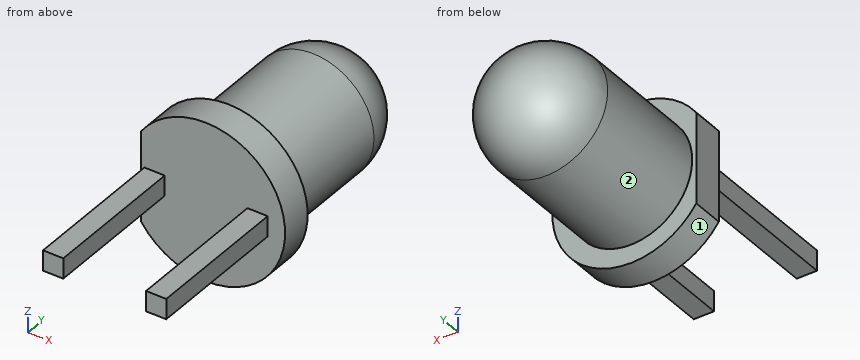
from build123d import *

# Parameters (mm, degrees)
ESQUISSE2_W             = 0.5
ESQUISSE2_H             = 0.5
BOSS_EXTRU_1_DEPTH      = 3.6
ESQUISSE3_W             = 1
ESQUISSE3_H             = 4
ENL_V_MAT_EXTRU_1_DEPTH = 6.3


with BuildPart() as part:
    # Esquisse1 → Révolution1 (revolve)
    with BuildSketch(Plane.XY):
        with BuildLine():
            Line((0, 0), (-1.95, 0))
            Line((-1.95, 0), (-1.95, 0.8))
            Line((-1.95, 0.8), (-1.5, 0.8))
            Line((-1.5, 0.8), (-1.5, 3.8))
            ThreePointArc((-1.5, 3.8), (-1.060660172, 4.860660172), (0, 5.3))
            Line((0, 5.3), (0, 0))
        make_face()
    revolve(axis=Axis((0, 5.3, 0), (0, -1, 0)))

    # Esquisse2 → Boss.-Extru.1 (add)
    with BuildSketch(Plane.XZ):
        with Locations((-1.27, 0)):
            Rectangle(ESQUISSE2_W, ESQUISSE2_H)
        with Locations((1.27, 0)):
            Rectangle(ESQUISSE2_W, ESQUISSE2_H)
    extrude(amount=BOSS_EXTRU_1_DEPTH)

    # Esquisse3 → Enlèv. mat.-Extru.1 (cut, through all)
    with BuildSketch(Plane.XZ):
        with Locations((-2.1, 0)):
            Rectangle(ESQUISSE3_W, ESQUISSE3_H)
    extrude(amount=-ENL_V_MAT_EXTRU_1_DEPTH, mode=Mode.SUBTRACT)


solid = part.part
The listing builds one solid part. Answer for the finished solid, in the listing's coordinates (mm). Face numbers are marked on the shaded views. A direction names the side the tool comes from. Coordinates: 2 decimals unless noted, no trailing zeros. Write each loop counter-clockwise with the first axis right and the second up, starting at its lowest first coordinate (ties: lowest second). Pieces come first, ordered by that corner, then holes. Notation, with made-up numbers: (-29, -28.75) - (27, -28.75) arc R18 ccw to (27, -10.75) - close; hole circle Ø5 at (45.25, 70.25). An arc over 180 degrees is marked (long way). Put each result on its own line as item: value.
1. A tool of negligible diameter and unlimited length cuts with its end or side. For the marked faces 1 and 2, from which of +Z, -Z, +X, -X, +Y, -Y can it reach the whole face along a straight path? Write none if from no direction.
Answer sheet:
face 1: +Y, -Y
face 2: +Y
2. Flat-ended cylindrical pins translate along their axes: pin 1 Ø0.6 at (x, y) = (-1.5, -1) entering from +Z; pin 2 Ø0.6 at (x, y) = (-1.5, -1) entering from -Z; pin 3 Ø0.6 at (y, z) = (-2.5, 0) entering from -X; pin 4 Ø1 at (y, z) = (-2, -1) entering from +X. Find the tip coordinate at first contact, or state that the pin passes through.
Answer sheet:
pin 1: stops at z = 0.25
pin 2: stops at z = -0.25
pin 3: stops at x = -1.52
pin 4: passes through
3. The part is cut by section D-D on x = -0.6. Give the vertices of the cut face in (y, z).
Answer sheet:
outline: (0, -1.86) - (0.8, -1.86) - (0.8, -1.37) - (3.8, -1.37) arc R1.37 ccw to (3.8, 1.37) - (0.8, 1.37) - (0.8, 1.86) - (0, 1.86) - close
4. The part is cut by section B-B on x = 0. Give the vertices of the cut face in (y, z).
Answer sheet:
outline: (0, -1.95) - (0.8, -1.95) - (0.8, -1.5) - (3.8, -1.5) arc R1.5 ccw to (3.8, 1.5) - (0.8, 1.5) - (0.8, 1.95) - (0, 1.95) - close
5. Find the intervals of material crossed by line 1 along X through (y, z) = (-1.75, 0.1); line 2 along Z through (x, y) = (1.35, -1.5); line 3 along Y through (x, z) = (1, -1.3), in increasing order. Write a range as from..to.
Answer sheet:
line 1: x = -1.52..-1.02, 1.02..1.52
line 2: z = -0.25..0.25
line 3: y = 0..0.8
6. The part is cut by section A-A on y = -1.25. Give the vertices of the cut face in (x, z), plus the area to 3 significant figures.
Answer sheet:
outline: (-1.52, -0.25) - (-1.02, -0.25) - (-1.02, 0.25) - (-1.52, 0.25) - close; (1.02, -0.25) - (1.52, -0.25) - (1.52, 0.25) - (1.02, 0.25) - close
area: 0.500 mm^2
7. The part is cut by section C-C on z = 0. Give the vertices of the cut face in (x, y).
Answer sheet:
outline: (-1.6, 0) - (-1.52, 0) - (-1.52, -3.6) - (-1.02, -3.6) - (-1.02, 0) - (1.02, 0) - (1.02, -3.6) - (1.52, -3.6) - (1.52, 0) - (1.95, 0) - (1.95, 0.8) - (1.5, 0.8) - (1.5, 3.8) arc R1.5 ccw to (-1.5, 3.8) - (-1.5, 0.8) - (-1.6, 0.8) - close
